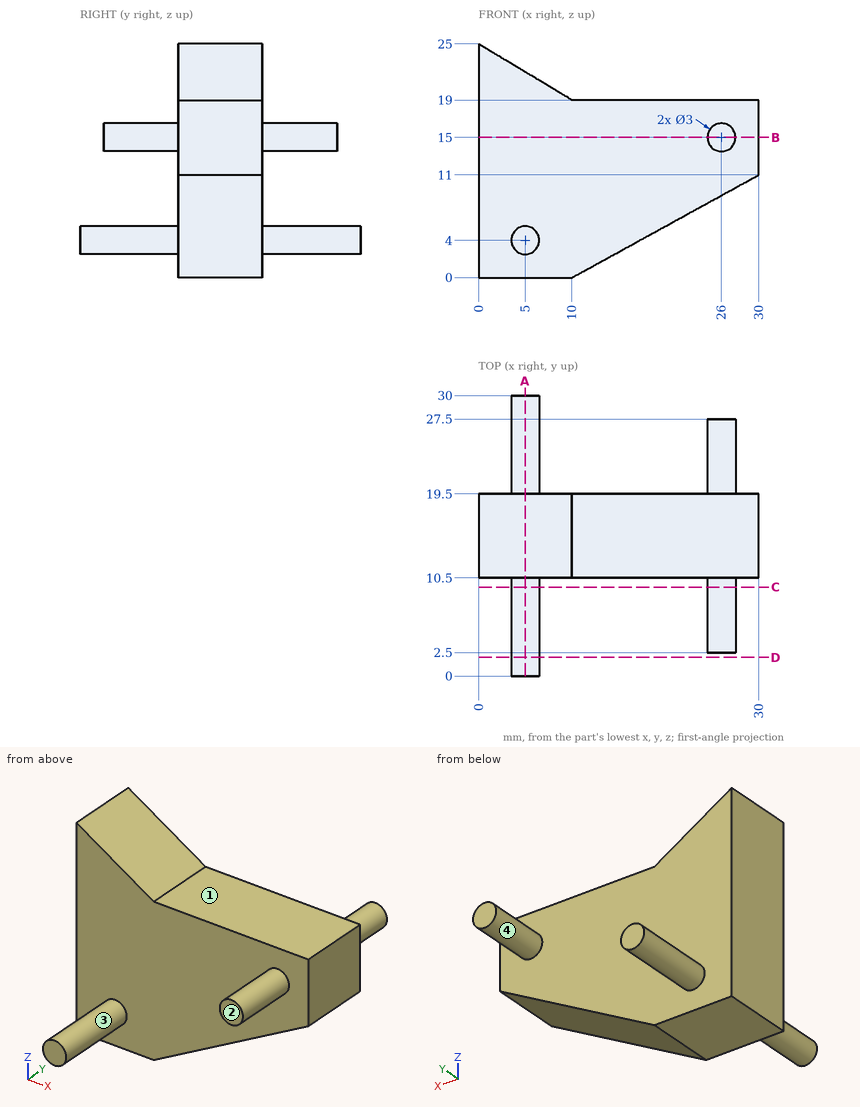
Verification items for this drawing (mm, ordinates from the low corner). A direction names the side the tool comes from. Coordinates: 2 decimals unless noted, no trailing zeros. Write each loop counter-clockwise with the first axis right and the second up, starting at its lowest first coordinate (ties: lowest second). Pieces come first, ordered by that corner, then holes. Notation, with made-up numbers: (56.5, -25.75) -> (100.5, -25.75) arc R23 ccw to (100.5, -4.75) -> close; hole circle Ø9 at (-16.75, -36.5). An arc over 180 degrees is marked (long way). One line per item, written item: value. Start each with the question number.
Q1. Access from +Z, -Z, +X, -X, +Y, -Y to the whole of each face (thin tool, end or side, straight path). Record for the marked faces 1, 2, 3 and 4.
Q2. Go/stop test with flat-tipped pins: P1, Ø1.5, axis at x = 25.5, z = 14.5, coming from the -Y side; P2, Ø10, axis at x = 16.5, z = 12, coming from the +Y side; P3, Ø5, axis at x = 6, z = 19, coming from the -Y side; P4, Ø8, axis at y = 10.5, z = 8, coming from the -X side. Record where each tip stops, or that it passes through.
Q3. Cross-section at A-A on x = 5. Enter the section's corners in (y, z).
Q4. Cross-section at D-D on y = 2. Enter the section's corners in (x, z), and give its area (3 significant figures).
Q5. Cross-section at C-C on y = 9.5. Enter the section's corners in (x, z).
Q6. Thickness scan on L1, parallel to Y at x = 26.5, z = 11; L2, parallel to X at y = 18.25, z = 8.5; L3, parallel to X at y = 13.5, z = 1. Record the ranges inside material, lowest first. Write a range as from..to.
Q7. Cross-section at B-B on z = 15. Enter the section's corners in (x, y).
Checked values:
1. face 1: +Z, +X, +Y, -Y
1. face 2: +Z, -Z, +X, -X, -Y
1. face 3: -Y
1. face 4: +Y
2. P1: stops at y = 2.5
2. P2: stops at y = 19.5
2. P3: stops at y = 10.5
2. P4: stops at x = 0
3. outline: (0, 2.5) -> (10.5, 2.5) -> (10.5, 0) -> (19.5, 0) -> (19.5, 2.5) -> (30, 2.5) -> (30, 5.5) -> (19.5, 5.5) -> (19.5, 22) -> (10.5, 22) -> (10.5, 5.5) -> (0, 5.5) -> close
4. outline: circle Ø3 at (5, 4)
4. area: 7.07 mm²
5. outline: circle Ø3 at (5, 4); circle Ø3 at (26, 15)
6. L1: y = 10.5..19.5
6. L2: x = 0..25.45
6. L3: x = 0..11.82
7. outline: (0, 10.5) -> (24.5, 10.5) -> (24.5, 2.5) -> (27.5, 2.5) -> (27.5, 10.5) -> (30, 10.5) -> (30, 19.5) -> (27.5, 19.5) -> (27.5, 27.5) -> (24.5, 27.5) -> (24.5, 19.5) -> (0, 19.5) -> close
